Can you work these out from the model? Positions are in its coordinate system, mm. A direction names the side the tool comes from. Round coordinates to 2 decimals unless told otherwise and drop trailing zeros. Order: outer loops, then holes, each group sorted by start corner. A loop starts at its lowest first (then second) coordinate and runs counter-clockwise, first axis right, second up.
from build123d import *

# Parameters (mm, degrees)
SKETCH_1_R            = 2.75
EXTRUDE_248_DEPTH     = 3
CUT_EXTRUDE_378_DEPTH = 1.3
SKETCH_3_R            = 1.5
EXTRUDE_479_DEPTH     = 14


with BuildPart() as part:
    # 草图1 → Extrude 248 (new body)
    with BuildSketch(Plane(origin=(0, 0, 0), x_dir=(1, 0, 0), z_dir=(0, 1, 0))):
        Circle(SKETCH_1_R)
    extrude(amount=EXTRUDE_248_DEPTH)

    # 草图2 → Cut-Extrude 378 (cut)
    with BuildSketch(Plane(origin=(0, 3, 0), x_dir=(1, 0, 0), z_dir=(0, 1, 0))):
        Polygon((1.443375673, 0), (0.721687836, 1.25), (-0.721687836, 1.25), (-1.443375673, 0), (-0.721687836, -1.25), (0.721687836, -1.25), align=None)
    extrude(amount=-CUT_EXTRUDE_378_DEPTH, mode=Mode.SUBTRACT)

    # 草图3 → Extrude 479 (add)
    with BuildSketch(Plane.XZ):
        Circle(SKETCH_3_R)
    extrude(amount=EXTRUDE_479_DEPTH)


solid = part.part
(1) I want a section at B-B, the plane z = -0.6. List the corners of the cut face in (x, y) for me, plus the area to 3 significant figures.
(2) Please list where these lines run through material, in increasing order: probe 1 along Y at (x, z) = (0.2, -0.15); probe 2 along Y at (x, z) = (0.9, 2.15); probe 3 along Z at (x, y) = (0, -10).
(3) I'm going to push flat-ended pins straight in: pin 1 Ø1 at (x, y) = (0.5, 2) entering from +Z; pin 2 Ø3 at (x, y) = (-0.5, -8.5) entering from -Z; pin 3 Ø2 at (y, z) = (-6, 2) entering from -X; pin 4 Ø3 at (y, z) = (-10, -1) entering from +X. Where does each tip first touch, or does it pass through?
(4) I want a section at C-C, the plane y = 1.5. List the corners of the cut face in (x, z) for me.
(5) I want a section at A-A, the plane x = 0. List the corners of the cut face in (y, z) for me, plus the area to 4 significant figures.
(6) On a 3-axis mill with a long thin cutter (end or side, diameter ignored), from which of +Z, -Z, +X, -X, +Y, -Y can I reach the whole of each face in a straight line? I mean faces 4 (the face through (0, 2, 1.25)), 5 (the face through (-0.596, 1.479, 2.685)). Say none if no direction works.
(7) If we mould it in two halves opening along Z, with no side actions, what happens to faces 1 (the face through (-1.5, -6.9, 0.07)), 2 (the face through (0, 2, -1.25)), 3 (the face through (1.2, 0, 1.2))? For each: pulls with the +Z half, pulls with the -Z half, needs draft (parallel to the pull), parting line crosses it, or undercut.
(8) I want a section at D-D, the plane x = 1.65. List the corners of the cut face in (y, z) for me.
Ans:
1. outline: (-2.68, 0) - (-1.37, 0) - (-1.37, -14) - (1.37, -14) - (1.37, 0) - (2.68, 0) - (2.68, 3) - (1.1, 3) - (1.1, 1.7) - (-1.1, 1.7) - (-1.1, 3) - (-2.68, 3) - close
1. area: 51.7 mm2
2. probe 1: y = -14 to 1.7
2. probe 2: y = 0 to 3
2. probe 3: z = -1.5 to 1.5
3. pin 1: stops at z = 2.75
3. pin 2: stops at z = -1.5
3. pin 3: stops at x = -1.12
3. pin 4: stops at x = 1.5
4. outline: circle Ø5.5 at (0, 0)
5. outline: (-14, -1.5) - (0, -1.5) - (0, -2.75) - (3, -2.75) - (3, -1.25) - (1.7, -1.25) - (1.7, 1.25) - (3, 1.25) - (3, 2.75) - (0, 2.75) - (0, 1.5) - (-14, 1.5) - close
5. area: 55.25 mm2
6. face 4: +Y
6. face 5: +Y, -Y
7. face 1: parting line crosses it
7. face 2: undercut
7. face 3: needs draft
8. outline: (0, -2.2) - (3, -2.2) - (3, 2.2) - (0, 2.2) - close
